```python
from build123d import *

# Parameters (mm, degrees)
SKETCH2_W           = 15.7
SKETCH2_H           = 82
BOSS_EXTRUDE1_DEPTH = 12
SKETCH3_W           = 8.7
SKETCH3_H           = 82
CUT_EXTRUDE1_DEPTH  = 10
SKETCH4_R           = 10.5
BOSS_EXTRUDE2_DEPTH = 12


with BuildPart() as part:
    # Sketch2 → Boss-Extrude1 (new body)
    with BuildSketch(Plane(origin=(0, 0, 0), x_dir=(1, 0, 0), z_dir=(0, 1, 0))):
        Rectangle(SKETCH2_W, SKETCH2_H)
    extrude(amount=BOSS_EXTRUDE1_DEPTH)

    # Sketch3 → Cut-Extrude1 (cut)
    with BuildSketch(Plane(origin=(0, 12, 0), x_dir=(1, 0, 0), z_dir=(0, 1, 0))):
        Rectangle(SKETCH3_W, SKETCH3_H)
    extrude(amount=-CUT_EXTRUDE1_DEPTH, mode=Mode.SUBTRACT)

    # Sketch4 → Boss-Extrude2 (add)
    with BuildSketch(Plane(origin=(0, 0, -41), x_dir=(-1, 0, 0), z_dir=(0, 0, -1))):
        with Locations((0, 6)):
            Circle(SKETCH4_R)
    extrude(amount=BOSS_EXTRUDE2_DEPTH)


solid = part.part
```
Geometry: final body of the model. Coordinates: model frame, mm. A direction names the side the tool comes from. Coordinates: 2 decimals unless noted, no trailing zeros. Order: outer loops, then holes, each group sorted by start corner. A loop starts at its lowest first (then second) coordinate and runs counter-clockwise, first axis right, second up. Notation, with made-up numbers: (84.25, -32.75) -> (125.25, -32.75) arc R34 cw to (125.25, 0.25) -> close; hole circle Ø8 at (32.5, -7). An arc over 180 degrees is marked (long way). Write item = value, one per line.
(1) Cut plane D-D on z = -46.5. Return loops of the section in (x, y), plus the area to 3 significant figures.
Solved:
outline = circle Ø21 at (0, 6)
area = 346 mm²
(2) Pin query (flat end, axial travel): pin 1 Ø3 at (x, z) = (-5.5, -10) entering from +Y; pin 2 Ø5 at (y, z) = (2, -34.5) entering from +X; pin 3 Ø1 at (x, z) = (7, -27) entering from -Y. Return the tip coordinate at first contact, or that it passes through.
Solved:
pin_1 = 12
pin_2 = 7.85
pin_3 = 0
(3) Cut plane C-C on y = 6. Return loops of the section in (x, z).
Solved:
outline = (-10.5, -53) -> (10.5, -53) -> (10.5, -41) -> (7.85, -41) -> (7.85, 41) -> (4.35, 41) -> (4.35, -41) -> (-4.35, -41) -> (-4.35, 41) -> (-7.85, 41) -> (-7.85, -41) -> (-10.5, -41) -> close
(4) Cut plane A-A on x = 0. Return loops of the section in (y, z).
Solved:
outline = (-4.5, -53) -> (16.5, -53) -> (16.5, -41) -> (2, -41) -> (2, 41) -> (0, 41) -> (0, -41) -> (-4.5, -41) -> close
(5) Line query: line 1 (X direction, y = 8.75, z = -17); line 2 (Z direction, x = 9, y = 1); line 3 (Y direction, x = -5.75, z = 7.5). Output: solid intervals per line, ascending.
Solved:
line_1 = -7.85 to -4.35, 4.35 to 7.85
line_2 = -53 to -41
line_3 = 0 to 12
(6) Pull-direction query (X, two-part tool) for faces 6 (the flat face through (7.85, 6, 1)), 7 (the flat face through (6, 12, -1)), 8 (the cylindrical face through (-4.845, -3.315, -46.916)), 9 (the flat face through (-4.35, 7, 1)); classes: pulls with the +X half, pulls with the -X half, needs draft (parallel to the pull), parting line crosses it, or undercut.
Solved:
face_6 = pulls with the +X half
face_7 = needs draft
face_8 = parting line crosses it
face_9 = undercut
(7) Cut plane B-B on z = -17. Return loops of the section in (x, y), plus the area to 3 significant figures.
Solved:
outline = (-7.85, 0) -> (7.85, 0) -> (7.85, 12) -> (4.35, 12) -> (4.35, 2) -> (-4.35, 2) -> (-4.35, 12) -> (-7.85, 12) -> close
area = 101 mm²
(8) Access query for faces 1 (the flat face through (-7.85, 6, 1)), 2 (the flat face through (0, 0, -1)), 3 (the flat face through (0, 2, -1)), 4 (the flat face through (0, 6, -53)), 5 (the flat face through (-6, 12, -1)). Directions: +Z, -Z, +X, -X, +Y, -Y. A direction counts if a zero-diameter tool reaches every point of the face in a straight line with its end or side. Return the directions, or none.
Solved:
face_1 = +Z, -X, +Y, -Y
face_2 = +Z, +X, -X, -Y
face_3 = +Z, +Y
face_4 = -Z, +X, -X, +Y, -Y
face_5 = +Z, +X, -X, +Y
